Check sheet for the modelled part. Datum: model origin and axes. Units: mm. Face numbers are marked on the shaded views. Round coordinates to 2 decimals unless told otherwise and drop trailing zeros. Loops run counter-clockwise (first coordinate to the right, second up) from the corner with the lowest first, then second, coordinate; pieces in that order, holes last. Notation, with made-up numbers: (80.5, 28) - (96.5, 28) arc R11 ccw to (96.5, 44) - close; hole circle Ø6 at (-12.5, 23). An arc over 180 degrees is marked (long way). Answer in a Markdown table with one row per item. Add a question column.
(1) Mould release check, pull along Z, two halves, no side actions. Record for the marked faces 1 and 2: +Z half, -Z half, draft (parallel to the pull), parting line (faces both ways), or undercut.
(2) Cross-section at A-A on x = -22.2. Enter the section's corners in (y, z).
(3) Cross-section at C-C on x = -7.5. Enter the section's corners in (y, z), then the cut area to 3 significant figures.
(4) Thickness scan on line 1 along Z through (x, y) = (-22.2, 0.8); line 2 along Z through (x, y) = (-22.2, 5.1); line 3 along X through (y, z) = (5.8, -48). Record the ranges inside material, lowest first.
(5) Cross-section at B-B on z = -48. Enter the section's corners in (x, y).
(6) Cross-section at D-D on z = 25. Enter the section's corners in (x, y).
(7) Gauge pin test, flat ends, axial feed: pin 1 (6.5 mm diameter, centred on x = -22.2, z = 48, fed in from +Y); pin 2 (2 mm diameter, centred on y = 1.5, z = 21.5, fed in from -X); pin 3 (12 mm diameter, centred on x = -22.5, z = 50, fed in from +Y); pin 4 (3.5 mm diameter, centred on x = -25, z = -49, fed in from +Y). Record the tip position at first contact, or that the pin passes through.
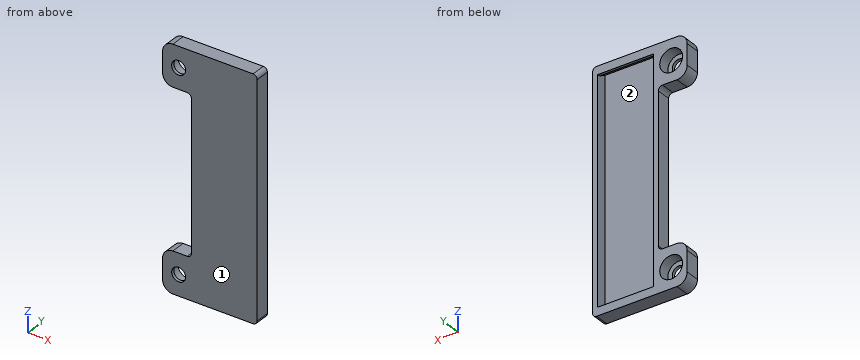
Autodesk Inventor part; units mm, degrees
ref_plane "YZ Plane" through (0, 0, 0) normal (1, 0, 0) x (0, 1, 0)
ref_plane "XZ Plane" through (0, 0, 0) normal (0, 1, 0) x (-1, 0, 0)
ref_plane "XY Plane" through (0, 0, 0) normal (0, 0, 1) x (1, 0, 0)
sketch "Sketch1" plane through (0, 0, 0) normal (0, 1, 0) x (-1, 0, 0)
  line L0 (-16, 58) -> (16, 58)
  line L1 (16, 58) -> (16, -58)
  line L2 (16, -58) -> (-16, -58)
  line L3 (-16, -58) -> (-16, 58)
  line L4 (-16, 58) -> (16, -58) construction
  line L5 (16, 58) -> (-16, -58) construction
  point P0 (0, 0)
  dimension "d0" = 32
  dimension "d1" = 116
extrude "Extrusion1" add sketch "Sketch1" along normal blind 7
sketch "Sketch3" plane through (16, 0, 58) normal (1, 0, 0) x (0, 0, -1)
  line L0 (0, 7) -> (116, 7)
  line L1 (4.75, 7) -> (1.8632, 2)
  line L2 (1.8632, 2) -> (114.1368, 2)
  line L3 (114.1368, 2) -> (111.25, 7)
  line L4 (0, 0) -> (0, 7)
  line L5 (116, 0) -> (116, 7)
  line L6 (4, 5.701) -> (4, 7)
  line L7 (116, 7) -> (0, 7)
  line L8 (112, 7) -> (112, 5.701)
  point P0 (58, 0)
  dimension "d4" = 60
  dimension "d6" = 60
  dimension "d7" = 5
  dimension "d8" = 106.5
  dimension "d9" = 116
  dimension "d10" = 4.75
  dimension "d17" = 4
  dimension "d18" = 4
extrude "Extrusion2" cut sketch "Sketch3" against normal through all
sketch "Sketch4" plane through (0, 7, 0) normal (0, 1, 0) x (1, 0, 0)
  line L0 (-16, 58) -> (-16, -58)
  line L1 (-16, -58) -> (-13.5, -58)
  line L2 (-13.5, -58) -> (-13.5, 58)
  line L3 (-13.5, 58) -> (-16, 58)
  line L4 (-16, 58) -> (-16, -58)
  line L5 (16, -58) -> (16, 58)
  line L6 (16, -58) -> (13.5, -58)
  line L7 (13.5, -58) -> (13.5, 58)
  line L8 (13.5, 58) -> (16, 58)
  line L9 (16, 58) -> (16, -58)
  line L10 (16, 58) -> (-16, 58)
  point P0 (0, 0)
  dimension "d13" = 2.5
  dimension "d14" = 2.5
extrude "Extrusion3" add sketch "Sketch4" against normal up to surface (7 mm away)
sketch "Sketch5" plane through (0, 7, 0) normal (0, 1, 0) x (1, 0, 0)
  line L0 (-16, 58) -> (-16, -58)
  line L1 (-16, -58) -> (-25, -58)
  line L2 (-30, -53) -> (-30, -43)
  line L3 (-25, -38) -> (-16, -38)
  line L4 (-16, -38) -> (-16, -58)
  arc A0 (-30, -53) -> (-25, -58) centre (-25, -53) ccw
  arc A1 (-25, -38) -> (-30, -43) centre (-25, -43) ccw
  line L5 (-36.8459, 0) -> (21.1314, 0)
  line L6 (-16, 58) -> (-25, 58)
  line L7 (-30, 53) -> (-30, 43)
  line L8 (-25, 38) -> (-16, 38)
  line L9 (-16, 38) -> (-16, 58)
  arc A2 (-25, 58) -> (-30, 53) centre (-25, 53) ccw
  arc A3 (-30, 43) -> (-25, 38) centre (-25, 43) ccw
  point P0 (0, 0)
  point P1 (-30, -38)
  point P2 (-30, -58)
  point P3 (-22.2, -48)
  point P4 (-30, 38)
  point P5 (-30, 58)
  point P6 (-22.2, 48)
  dimension "d19" = 20
  dimension "d20" = 14
  dimension "d21" = 22.2
  dimension "d22" = 10
  dimension "d23" = 6.2
  dimension "d33" = 5
extrude "Extrusion4" add sketch "Sketch5" against normal up to surface (7 mm away)
hole "Hole1" at (-22.2, 7, 48) at (-22.2, 7, -48) direction (0, -1, 0) diameter 6.756 depth 19.05 tip angle 118 counterbore diameter 11.113 counterbore depth 5.5
fillet "Fillet1" radius 2 4 edges at (16, 3.5, -58) (16, 3.5, 58) (-16, 3.5, 38) (-16, 3.5, -38)
equation "\"d10\" = -0.5 * d8 + 0.5 * d9"
properties part number "Bracket Clamp"
Answers:
| question | item | result |
|---|---|---|
| 1 | face 1 | draft |
| 1 | face 2 | undercut |
| 2 | outline | (0, -58) - (7, -58) - (7, -53.56) - (1.5, -53.56) - (1.5, -51.38) - (0, -51.38) - close; (0, -44.62) - (1.5, -44.62) - (1.5, -42.44) - (7, -42.44) - (7, -38) - (0, -38) - close; (0, 38) - (7, 38) - (7, 42.44) - (1.5, 42.44) - (1.5, 44.62) - (0, 44.62) - close; (0, 51.38) - (1.5, 51.38) - (1.5, 53.56) - (7, 53.56) - (7, 58) - (0, 58) - close |
| 3 | outline | (0, -58) - (7, -58) - (7, -54) - (5.7, -54) - (2, -56.14) - (2, 56.14) - (5.7, 54) - (7, 54) - (7, 58) - (0, 58) - close |
| 3 | area | 264 mm^2 |
| 4 | line 1 | z = -58 to -51.38, -44.62 to -38, 38 to 44.62, 51.38 to 58 |
| 4 | line 2 | z = -58 to -53.56, -42.44 to -38, 38 to 42.44, 53.56 to 58 |
| 4 | line 3 | x = -30 to -27.76, -16.64 to -13.5, 13.5 to 16 |
| 5 | outline | (-30, 0) - (-25.58, 0) - (-25.58, 1.5) - (-27.76, 1.5) - (-27.76, 7) - (-30, 7) - close; (-18.82, 0) - (16, 0) - (16, 7) - (13.5, 7) - (13.5, 2) - (-13.5, 2) - (-13.5, 7) - (-16.64, 7) - (-16.64, 1.5) - (-18.82, 1.5) - close |
| 6 | outline | (-16, 0) - (16, 0) - (16, 7) - (13.5, 7) - (13.5, 2) - (-13.5, 2) - (-13.5, 7) - (-16, 7) - close |
| 7 | pin 1 | passes through |
| 7 | pin 2 | stops at x = -16 |
| 7 | pin 3 | stops at y = 7 |
| 7 | pin 4 | stops at y = 1.5 |
